The listing builds one solid part. Answer for the finished solid, in the listing's coordinates (mm). Round coordinates to 2 decimals unless told otherwise and drop trailing zeros. Order: outer loops, then holes, each group sorted by start corner. A loop starts at its lowest first (then second) coordinate and runs counter-clockwise, first axis right, second up. Notation, with made-up numbers: M 62,55.5 L 103,55.5 A25 ccw 103,82.5 Z; hole C 40,12.25 d6. An arc over 180 degrees is marked long. Write item = value, one per line. Start each with the question number.
(1) Each of these flat-tipped pins is pushed along its axis until it touches: pin 1 (6 mm diameter, centred on y = 132.5, z = -7.5, fed in from +X); pin 2 (2 mm diameter, centred on y = 131, z = -3.5, fed in from -X); pin 3 (3 mm diameter, centred on x = 21, y = 6.5, fed in from -Z). Where does it stop, or does it pass through?
(2) A cutting plane is placed at A-A, the plane z = -11.25. Determine the outline of the cut face in (x, y), and give its area (3 significant figures).
(3) A cutting plane is placed at B-B, the plane y = 151.5. Determine the outline of the cut face in (x, z), and give its area (3 significant figures).
(4) A cutting plane is placed at C-C, the plane x = 96. Determine the outline of the cut face in (y, z).
(5) A straight line is drawn through the part: probe 1 along Z at (x, y) = (22, 109.5). Find the intervals that lie inside material, in ascending order. Write a range as from..to.
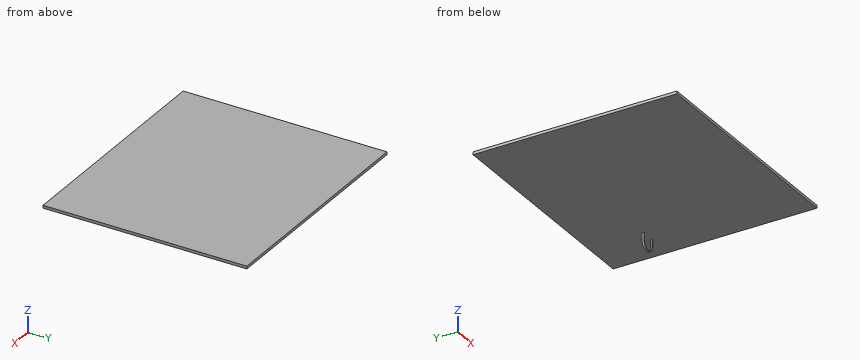
from build123d import *

# Parameters (mm, degrees)
SKETCH1_W           = 250
SKETCH1_H           = 220
BOSS_EXTRUDE1_DEPTH = 3
EXTRUDE_THIN1_DEPTH = 2


with BuildPart() as part:
    # Sketch1 → Boss-Extrude1 (new body)
    with BuildSketch(Plane.XY):
        with Locations((35.461157826, 79.854863969)):
            Rectangle(SKETCH1_W, SKETCH1_H)
    extrude(amount=BOSS_EXTRUDE1_DEPTH)

    # Sketch2 → Extrude-Thin1 (add)
    with BuildSketch(Plane(origin=(0, 129.854863969, 0), x_dir=(1, 0, 0), z_dir=(0, 1, 0))):
        with BuildLine():
            ThreePointArc((117.298879334, 7.909094463), (123.99586371, 15.093149798), (131.021373602, 8.230026488))
            Line((131.021373602, 8.230026488), (131.021373602, 0))
            Line((131.021373602, 0), (132.021373602, 0))
            Line((132.021373602, 0), (132.021373602, 8.230026488))
            ThreePointArc((132.021373602, 8.230026488), (123.972482809, 16.092876428), (116.299972667, 7.862345443))
            Line((116.299972667, 7.862345443), (117.298879334, 7.909094463))
        make_face()
        Polygon((117.483851661, 0), (117.291373602, 8.230026488), (116.291646972, 8.206645586), (116.484125031, -0.023380902), align=None)
    extrude(amount=EXTRUDE_THIN1_DEPTH)


solid = part.part
Reported:
q1.pin_1 = 132.02
q1.pin_2 = 116.38
q1.pin_3 = 0
q2.outline = M 116.89,129.85 L 117.99,129.85 L 117.99,131.85 L 116.89,131.85 Z; M 130.32,129.85 L 131.42,129.85 L 131.42,131.85 L 130.32,131.85 Z
q2.area = 4.39 mm²
q3.outline = M -89.54,0 L 160.46,0 L 160.46,3 L -89.54,3 Z
q3.area = 750 mm²
q4.outline = M -30.15,0 L 189.85,0 L 189.85,3 L -30.15,3 Z
q5.probe_1 = 0..3
